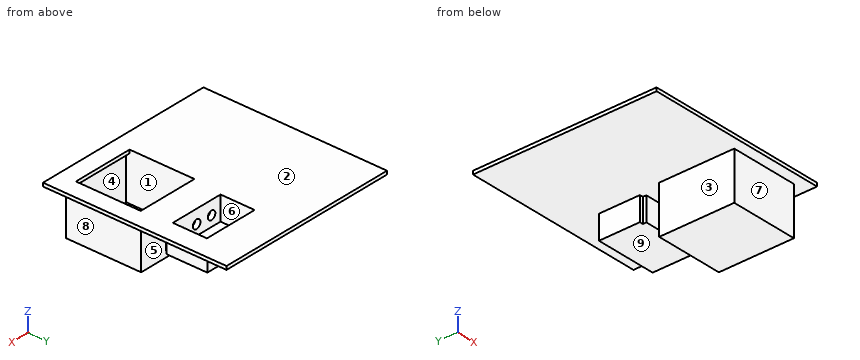
from build123d import *

# Parameters (mm, degrees)
SKETCH1_W           = 683.26
SKETCH1_H           = 683.26
SKETCH1_W_2         = 203.2
SKETCH1_H_2         = 127
BOSS_EXTRUDE1_DEPTH = 12.7
SKETCH2_W           = 203.2
SKETCH2_H           = 76.2
BOSS_EXTRUDE2_DEPTH = 25.4
SKETCH3_R           = 16.0655
CUT_EXTRUDE1_DEPTH  = 19.05
SKETCH4_W           = 12.7
SKETCH4_H           = 12.7
SKETCH4_H_2         = 127
SKETCH4_W_2         = 203.2
BOSS_EXTRUDE4_DEPTH = 76.2
BOSS_EXTRUDE5_DEPTH = 12.7
SKETCH6_W           = 228.6
SKETCH6_H           = 254
CUT_EXTRUDE2_DEPTH  = 972.60229271
SKETCH7_W           = 228.6
SKETCH7_H           = 12.7
BOSS_EXTRUDE6_DEPTH = 177.8
SKETCH8_W           = 12.7
SKETCH8_H           = 279.4
BOSS_EXTRUDE7_DEPTH = 177.8
SKETCH9_W           = 228.6
SKETCH9_H           = 12.7
BOSS_EXTRUDE8_DEPTH = 254
SKETCH10_W          = 228.6
SKETCH10_H          = 12.7
BOSS_EXTRUDE9_DEPTH = 12.7


with BuildPart() as part:
    # Sketch1 → Boss-Extrude1 (new body)
    with BuildSketch(Plane.XY):
        with Locations((341.63, 341.63)):
            Rectangle(SKETCH1_W, SKETCH1_H)
        with Locations((505.46, 480.06)):
            Rectangle(SKETCH1_W_2, SKETCH1_H_2, mode=Mode.SUBTRACT)
    extrude(amount=BOSS_EXTRUDE1_DEPTH)

    # Sketch2 → Boss-Extrude2 (add)
    with BuildSketch(Plane(origin=(0, 416.56, 0), x_dir=(1, 0, 0), z_dir=(0, 1, 0))):
        with Locations((505.46, 38.1)):
            Rectangle(SKETCH2_W, SKETCH2_H)
    extrude(amount=-BOSS_EXTRUDE2_DEPTH)

    # Sketch3 → Cut-Extrude1 (cut)
    with BuildSketch(Plane(origin=(0, 416.56, 0), x_dir=(1, 0, 0), z_dir=(0, 1, 0))):
        with Locations(Location((568.96, 38.1, 0), (0, 0, 270))):
            Circle(SKETCH3_R)
        with Locations(Location((505.46, 38.1, 0), (0, 0, 270))):
            Circle(SKETCH3_R)
        with Locations(Location((441.96, 38.1, 0), (0, 0, 270))):
            Circle(SKETCH3_R)
    extrude(amount=-CUT_EXTRUDE1_DEPTH, mode=Mode.SUBTRACT)

    # Sketch4 → Boss-Extrude4 (add)
    with BuildSketch(Plane(origin=(0, 0, 0), x_dir=(-1, 0, 0), z_dir=(0, 0, -1))):
        with Locations((-613.41, 410.21)):
            Rectangle(SKETCH4_W, SKETCH4_H)
        with Locations((-613.41, 480.06)):
            Rectangle(SKETCH4_W, SKETCH4_H_2)
        with Locations((-505.46, 549.91)):
            Rectangle(SKETCH4_W_2, SKETCH4_H)
        with Locations((-613.41, 549.91)):
            Rectangle(SKETCH4_W, SKETCH4_H)
        with Locations((-397.51, 549.91)):
            Rectangle(SKETCH4_W, SKETCH4_H)
        with Locations((-397.51, 480.06)):
            Rectangle(SKETCH4_W, SKETCH4_H_2)
        with Locations((-397.51, 410.21)):
            Rectangle(SKETCH4_W, SKETCH4_H)
    extrude(amount=BOSS_EXTRUDE4_DEPTH)

    # Sketch5 → Boss-Extrude5 (add)
    with BuildSketch(Plane(origin=(0, 0, -76.2), x_dir=(-1, 0, 0), z_dir=(0, 0, -1))):
        Polygon((-607.06, 391.16), (-403.86, 391.16), (-403.86, 403.86), (-391.16, 403.86), (-391.16, 556.26), (-619.76, 556.26), (-619.76, 403.86), (-607.06, 403.86), align=None)
    extrude(amount=BOSS_EXTRUDE5_DEPTH)

    # Sketch6 → Cut-Extrude2 (cut, through all)
    with BuildSketch(Plane.XY.offset(12.7)):
        with Locations((503.315588228, 179.399098269)):
            Rectangle(SKETCH6_W, SKETCH6_H)
    extrude(amount=-CUT_EXTRUDE2_DEPTH, mode=Mode.SUBTRACT)

    # Sketch7 → Boss-Extrude6 (add)
    with BuildSketch(Plane(origin=(0, 0, 0), x_dir=(-1, 0, 0), z_dir=(0, 0, -1))):
        with Locations((-503.315588228, 46.049098269)):
            Rectangle(SKETCH7_W, SKETCH7_H)
    boss_extrude6 = extrude(amount=BOSS_EXTRUDE6_DEPTH)

    # Mirror1: Boss-Extrude6 across plane
    add(boss_extrude6.mirror(Plane.ZX.offset(179.399098269)))

    # Sketch8 → Boss-Extrude7 (add)
    with BuildSketch(Plane(origin=(0, 0, 0), x_dir=(-1, 0, 0), z_dir=(0, 0, -1))):
        with Locations((-623.965588228, 179.399098269)):
            Rectangle(SKETCH8_W, SKETCH8_H)
        with Locations((-382.665588228, 179.399098269)):
            Rectangle(SKETCH8_W, SKETCH8_H)
    extrude(amount=BOSS_EXTRUDE7_DEPTH)

    # Sketch9 → Boss-Extrude8 (add)
    with BuildSketch(Plane(origin=(0, 52.399098269, 0), x_dir=(1, 0, 0), z_dir=(0, 1, 0))):
        with Locations((503.315588228, 171.45)):
            Rectangle(SKETCH9_W, SKETCH9_H)
    extrude(amount=BOSS_EXTRUDE8_DEPTH)

    # Sketch10 → Boss-Extrude9 (add)
    with BuildSketch(Plane(origin=(0, 52.399098269, 0), x_dir=(1, 0, 0), z_dir=(0, 1, 0))):
        with Locations((503.315588228, -6.35)):
            Rectangle(SKETCH10_W, SKETCH10_H)
    extrude(amount=BOSS_EXTRUDE9_DEPTH)


solid = part.part
Here's how the part is built. I have some questions about the finished solid (model axes, mm). Face numbers are marked on the shaded views. A direction names the side the tool comes from. Give positions to 0.01 mm unless a question says otherwise; leave off trailing zeros. Loops run counter-clockwise (first coordinate to the right, second up) from the corner with the lowest first, then second, coordinate; pieces in that order, holes last. Notation, with made-up numbers: (50, -37) -> (69, -37) arc R16 ccw to (69, -32) -> close; hole circle Ø1 at (15.5, -6.75). An arc over 180 degrees is marked (long way). Answer as a JSON object with one key per item and string values. Group by question number.
Item 1: Imagine slicing it at D-D on y = 432.5. Write out the boundary of the cut face in (x, z).
Item 2: Imagine slicing it at C-C on y = 170. Write out the boundary of the cut face in (x, z).
Item 3: Thinking about a two-plate mould opening in X: for the marked faces 1, 2, 3 and 4, which applies, pulls with the +X half, pulls with the -X half, needs draft (parallel to the pull), parting line crosses it, or undercut?
Item 4: On a 3-axis mill with a long thin cutter (end or side, diameter ignored), from which of +Z, -Z, +X, -X, +Y, -Y can I reach the whole of each face in a straight line? I mean the marked faces 5, 6, 7, 8 and 9. Say none if no direction works.
Item 5: Will these pins go through, and if not, where does the flat tip stop? pin 1 (1.5 mm diameter, centred on x = 317.5, y = 543, fed in from -Z); pin 2 (16 mm diameter, centred on x = 443.5, z = -35, fed in from +Y); pin 3 (1 mm diameter, centred on y = 442, z = -18.5, fed in from +X).
Item 6: Imagine slicing it at B-B on x = 568.96. Write out the boundary of the cut face in (y, z).
Item 7: Imagine slicing it at A-A on z = -38.1. Give the number of separate pieces and of enclosed holes in the cut face, then the cut area to 3 significant figures.
Item 8: I need wall thicknesses on L1, parallel to X at y = 402, z = -38.1; L2, parallel to Y at x = 465.5, z = -86; L3, parallel to X at y = 404, z = -38.1. Which ranges of each line are inside material? Lowest first, please.
Answer list:
{
 "1": {"outline": "(0, 0) -> (391.16, 0) -> (391.16, -88.9) -> (619.76, -88.9) -> (619.76, 0) -> (683.26, 0) -> (683.26, 12.7) -> (607.06, 12.7) -> (607.06, -76.2) -> (403.86, -76.2) -> (403.86, 12.7) -> (0, 12.7) -> close"},
 "2": {"outline": "(0, 0) -> (376.32, 0) -> (376.32, -177.8) -> (630.32, -177.8) -> (630.32, 0) -> (683.26, 0) -> (683.26, 12.7) -> (617.62, 12.7) -> (617.62, -165.1) -> (389.02, -165.1) -> (389.02, 12.7) -> (0, 12.7) -> close"},
 "3": {"face 1": "undercut", "face 2": "needs draft", "face 3": "pulls with the -X half", "face 4": "undercut"},
 "4": {"face 5": "-Z, +X, -X", "face 6": "+Z", "face 7": "-Z, +X, -X, -Y", "face 8": "-Z, +X, +Y, -Y", "face 9": "-Z, +X, -X, +Y"},
 "5": {"pin 1": "stops at z = 0", "pin 2": "stops at y = 556.26", "pin 3": "stops at x = 619.76"},
 "6": {"outline": "(0, 0) -> (39.7, 0) -> (39.7, -177.8) -> (319.1, -177.8) -> (319.1, 0) -> (391.16, 0) -> (391.16, -88.9) -> (556.26, -88.9) -> (556.26, 0) -> (683.26, 0) -> (683.26, 12.7) -> (543.56, 12.7) -> (543.56, -76.2) -> (416.56, -76.2) -> (416.56, -54.17) -> (397.51, -54.17) -> (397.51, -22.03) -> (416.56, -22.03) -> (416.56, 12.7) -> (306.4, 12.7) -> (306.4, -165.1) -> (52.4, -165.1) -> (52.4, 0) -> (65.1, 0) -> (65.1, 12.7) -> (0, 12.7) -> close"},
 "7": {"separate pieces": "2", "enclosed holes": "2", "area": "22,700 mm2"},
 "8": {"L1": "x = 403.86 to 425.89, 458.03 to 489.39, 521.53 to 552.89, 585.03 to 607.06", "L2": "y = 39.7 to 52.4, 306.4 to 319.1, 391.16 to 556.26", "L3": "x = 391.16 to 425.89, 458.03 to 489.39, 521.53 to 552.89, 585.03 to 619.76"}
}
